Could you check a few things on this model? Use its own coordinates, in mm. A direction names the side the tool comes from. Give positions to 0.01 mm unless a question says otherwise; leave off trailing zeros. Order: outer loops, then holes, each group sorted by start corner. A loop starts at its lowest first (then second) coordinate and runs counter-clockwise, first axis right, second up. Notation, with made-up numbers: (-33, -17.5) -> (-25, -17.5) arc R26 ccw to (-25, -0.5) -> close; hole circle Ø2 at (77, 13.5). An arc over 180 degrees is marked (long way). Answer as CSV lines item,"result". Start each with the question number.
(1) Will these pins go through, and if not, where does the flat tip stop? pin 1 Ø10 at (x, y) = (-2.5, -11) entering from -Z; pin 2 Ø7 at (x, y) = (3, 9.5) entering from +Z; pin 3 Ø3 at (x, y) = (2, -9) entering from -Z; pin 4 Ø1.5 at (x, z) = (0.5, 11.5) entering from -Y.
(2) On a 3-axis mill with a long thin cutter (end or side, diameter ignored), from which of +Z, -Z, +X, -X, +Y, -Y can I reach the whole of each face in a straight line? I mean faces 4 (the face through (-7.75, 8.94, 4.56)), 5 (the face through (0, -11, 8)), 6 (the face through (-11.5, 8.9, 14.6)), 7 (the face through (0.1, -6.5, 15)), 8 (the face through (0, 16, 10)). Say none if no direction works.
(3) I want a section at C-C (z = 12.5). Please give me the cut outline in (x, y).
(4) I want a section at A-A (x = 0). Give the number of separate pieces and of enclosed holes in the cut face, plus the area to 3 significant figures.
(5) We'd pull the mould along X, two halves only. Please class faces 1 (the face through (-12.215, -15.699, 9.874)), 2 (the face through (0, 4.5, 15)), 3 (the face through (0, 0, 0)): released by +X, released by -X, zero draft, split by the parting line, or undercut.
(6) I want a section at D-D (y = -10). Please give me the cut outline in (x, z).
(7) I need wall thicknesses on L1, parallel to Y at x = 2.25, z = 6.5; L2, parallel to Y at x = 7, z = 18.5; L3, parallel to Y at x = 9.5, z = 10.25. Which ranges of each line are inside material? Lowest first, please.
(8) I want a section at B-B (y = 9). Please give me the cut outline in (x, z), plus the area to 3 significant figures.
```python
from build123d import *

# Parameters (mm, degrees)
CROQUIS1_W              = 25
CROQUIS1_H              = 32
SALIENTE_EXTRUIR1_DEPTH = 20
CORTAR_EXTRUIR2_DEPTH   = 20
CORTAR_EXTRUIR3_DEPTH   = 10
CROQUIS9_R              = 2.5
CORTAR_EXTRUIR4_DEPTH   = 10
CROQUIS10_W             = 8
CROQUIS10_H             = 4
CORTAR_EXTRUIR5_DEPTH   = 17
REDONDEO1_R             = 1


with BuildPart() as part:
    # Croquis1 → Saliente-Extruir1 (new body)
    with BuildSketch(Plane.XY):
        Rectangle(CROQUIS1_W, CROQUIS1_H)
    extrude(amount=SALIENTE_EXTRUIR1_DEPTH)

    # Croquis7 → Cortar-Extruir2 (cut)
    with BuildSketch(Plane.XY.offset(20)):
        with BuildLine():
            Line((-5, 11.75), (5, 11.75))
            ThreePointArc((5, 11.75), (7.75, 9), (5, 6.25))
            Line((5, 6.25), (-5, 6.25))
            ThreePointArc((-5, 6.25), (-7.75, 9), (-5, 11.75))
        make_face()
    extrude(amount=-CORTAR_EXTRUIR2_DEPTH, mode=Mode.SUBTRACT)

    # Croquis8 → Cortar-Extruir3 (cut)
    with BuildSketch(Plane.XY.offset(20)):
        with BuildLine():
            Line((-7, 13.5), (7, 13.5))
            ThreePointArc((7, 13.5), (11.5, 9), (7, 4.5))
            Line((7, 4.5), (-7, 4.5))
            ThreePointArc((-7, 4.5), (-11.5, 9), (-7, 13.5))
        make_face()
    extrude(amount=-CORTAR_EXTRUIR3_DEPTH, mode=Mode.SUBTRACT)

    # Croquis9 → Cortar-Extruir4 (cut)
    with BuildSketch(Plane.XZ.offset(16)):
        with Locations(Location((0, 12.5, 0), (0, 0, 270))):
            Circle(CROQUIS9_R)
    extrude(amount=-CORTAR_EXTRUIR4_DEPTH, mode=Mode.SUBTRACT)

    # Croquis10 → Cortar-Extruir5 (cut)
    with BuildSketch(Plane(origin=(0, 0, 0), x_dir=(-1, 0, 0), z_dir=(0, 0, -1))):
        with Locations((0, -9)):
            Rectangle(CROQUIS10_W, CROQUIS10_H)
    extrude(amount=-CORTAR_EXTRUIR5_DEPTH, mode=Mode.SUBTRACT)

    # Redondeo1
    # the kernel refuses this fillet: 1 mm, written as the material it takes off along each edge
    with BuildSketch(Plane(origin=(11.5, -15, 19), x_dir=(0, 0, 1), z_dir=(1, 0, 0))) as redondeo1_piece_1_section:
        Polygon((0, 0), (REDONDEO1_R, 0), (REDONDEO1_R, REDONDEO1_R), (0, REDONDEO1_R), align=None)
    redondeo1_piece_1 = extrude(amount=REDONDEO1_R, mode=Mode.PRIVATE)
    redondeo1_piece_1 = redondeo1_piece_1 - Plane(origin=(11.5, -15, 19), x_dir=(0, 0.7071067811865475, -0.7071067811865475), z_dir=(1, 0, 0)) * Sphere(REDONDEO1_R, mode=Mode.PRIVATE)
    add(redondeo1_piece_1, mode=Mode.SUBTRACT)
    with BuildSketch(Plane(origin=(11.5, 15, 19), x_dir=(1, 0, 0), z_dir=(0, 1, 0))) as redondeo1_piece_2_section:
        Polygon((0, 0), (REDONDEO1_R, 0), (REDONDEO1_R, -REDONDEO1_R), (0, -REDONDEO1_R), align=None)
    redondeo1_piece_2 = extrude(amount=REDONDEO1_R, mode=Mode.PRIVATE)
    redondeo1_piece_2 = redondeo1_piece_2 - Plane(origin=(11.5, 15, 19), x_dir=(-0.7071067811865475, 0, -0.7071067811865475), z_dir=(0, 1, 0)) * Sphere(REDONDEO1_R, mode=Mode.PRIVATE)
    add(redondeo1_piece_2, mode=Mode.SUBTRACT)
    with BuildSketch(Plane(origin=(-11.5, 15, 19), x_dir=(-1, 0, 0), z_dir=(0, 1, 0))) as redondeo1_piece_3_section:
        Polygon((0, 0), (REDONDEO1_R, 0), (REDONDEO1_R, REDONDEO1_R), (0, REDONDEO1_R), align=None)
    redondeo1_piece_3 = extrude(amount=REDONDEO1_R, mode=Mode.PRIVATE)
    redondeo1_piece_3 = redondeo1_piece_3 - Plane(origin=(-11.5, 15, 19), x_dir=(0.7071067811865475, 0, -0.7071067811865475), z_dir=(0, 1, 0)) * Sphere(REDONDEO1_R, mode=Mode.PRIVATE)
    add(redondeo1_piece_3, mode=Mode.SUBTRACT)
    with BuildSketch(Plane(origin=(-11.5, -15, 19), x_dir=(0, 0, 1), z_dir=(-1, 0, 0))) as redondeo1_piece_4_section:
        Polygon((0, 0), (REDONDEO1_R, 0), (REDONDEO1_R, -REDONDEO1_R), (0, -REDONDEO1_R), align=None)
    redondeo1_piece_4 = extrude(amount=REDONDEO1_R, mode=Mode.PRIVATE)
    redondeo1_piece_4 = redondeo1_piece_4 - Plane(origin=(-11.5, -15, 19), x_dir=(0, 0.7071067811865475, -0.7071067811865475), z_dir=(-1, 0, 0)) * Sphere(REDONDEO1_R, mode=Mode.PRIVATE)
    add(redondeo1_piece_4, mode=Mode.SUBTRACT)
    with BuildSketch(Plane(origin=(11.5, 15, 1), x_dir=(1, 0, 0), z_dir=(0, 1, 0))) as redondeo1_piece_5_section:
        Polygon((0, 0), (REDONDEO1_R, 0), (REDONDEO1_R, REDONDEO1_R), (0, REDONDEO1_R), align=None)
    redondeo1_piece_5 = extrude(amount=REDONDEO1_R, mode=Mode.PRIVATE)
    redondeo1_piece_5 = redondeo1_piece_5 - Plane(origin=(11.5, 15, 1), x_dir=(-0.7071067811865475, 0, 0.7071067811865475), z_dir=(0, 1, 0)) * Sphere(REDONDEO1_R, mode=Mode.PRIVATE)
    add(redondeo1_piece_5, mode=Mode.SUBTRACT)
    with BuildSketch(Plane(origin=(-11.5, 15, 1), x_dir=(-1, 0, 0), z_dir=(0, 1, 0))) as redondeo1_piece_6_section:
        Polygon((0, 0), (REDONDEO1_R, 0), (REDONDEO1_R, -REDONDEO1_R), (0, -REDONDEO1_R), align=None)
    redondeo1_piece_6 = extrude(amount=REDONDEO1_R, mode=Mode.PRIVATE)
    redondeo1_piece_6 = redondeo1_piece_6 - Plane(origin=(-11.5, 15, 1), x_dir=(0.7071067811865475, 0, 0.7071067811865475), z_dir=(0, 1, 0)) * Sphere(REDONDEO1_R, mode=Mode.PRIVATE)
    add(redondeo1_piece_6, mode=Mode.SUBTRACT)
    with BuildSketch(Plane(origin=(11.5, -15, 1), x_dir=(0, 0, -1), z_dir=(1, 0, 0))) as redondeo1_piece_7_section:
        Polygon((0, 0), (REDONDEO1_R, 0), (REDONDEO1_R, -REDONDEO1_R), (0, -REDONDEO1_R), align=None)
    redondeo1_piece_7 = extrude(amount=REDONDEO1_R, mode=Mode.PRIVATE)
    redondeo1_piece_7 = redondeo1_piece_7 - Plane(origin=(11.5, -15, 1), x_dir=(0, 0.7071067811865475, 0.7071067811865475), z_dir=(1, 0, 0)) * Sphere(REDONDEO1_R, mode=Mode.PRIVATE)
    add(redondeo1_piece_7, mode=Mode.SUBTRACT)
    with BuildSketch(Plane(origin=(-11.5, -15, 1), x_dir=(0, 0, -1), z_dir=(-1, 0, 0))) as redondeo1_piece_8_section:
        Polygon((0, 0), (REDONDEO1_R, 0), (REDONDEO1_R, REDONDEO1_R), (0, REDONDEO1_R), align=None)
    redondeo1_piece_8 = extrude(amount=REDONDEO1_R, mode=Mode.PRIVATE)
    redondeo1_piece_8 = redondeo1_piece_8 - Plane(origin=(-11.5, -15, 1), x_dir=(0, 0.7071067811865475, 0.7071067811865475), z_dir=(-1, 0, 0)) * Sphere(REDONDEO1_R, mode=Mode.PRIVATE)
    add(redondeo1_piece_8, mode=Mode.SUBTRACT)
    with BuildSketch(Plane(origin=(12.5, -15, 20), x_dir=(0, 0, -1), z_dir=(0, 1, 0)), Plane(origin=(-12.5, 15, 20), x_dir=(0, 0, -1), z_dir=(0, -1, 0))) as redondeo1_piece_9:
        with BuildLine():
            CenterArc((REDONDEO1_R, REDONDEO1_R), REDONDEO1_R, 180, 90)
            Line((0, REDONDEO1_R), (0, 0))
            Line((0, 0), (REDONDEO1_R, 0))
        make_face()
    extrude(amount=30, mode=Mode.SUBTRACT)
    with BuildSketch(Plane(origin=(11.5, 16, 20), x_dir=(0, 0, -1), z_dir=(-1, 0, 0)), Plane(origin=(-11.5, -16, 0), x_dir=(0, 1, 0), z_dir=(1, 0, 0))) as redondeo1_piece_10:
        with BuildLine():
            CenterArc((REDONDEO1_R, REDONDEO1_R), REDONDEO1_R, 180, 90)
            Line((0, REDONDEO1_R), (0, 0))
            Line((0, 0), (REDONDEO1_R, 0))
        make_face()
    extrude(amount=23, mode=Mode.SUBTRACT)
    with BuildSketch(Plane(origin=(5, 6.25, 10), x_dir=(0, 0, -1), z_dir=(-1, 0, 0)), Plane(origin=(-5, 11.75, 10), x_dir=(0, 0, -1), z_dir=(1, 0, 0))) as redondeo1_piece_11:
        with BuildLine():
            CenterArc((REDONDEO1_R, REDONDEO1_R), REDONDEO1_R, 180, 90)
            Line((0, REDONDEO1_R), (0, 0))
            Line((0, 0), (REDONDEO1_R, 0))
        make_face()
    extrude(amount=10, mode=Mode.SUBTRACT)
    with BuildSketch(Plane(origin=(-7, 9, 20), x_dir=(0, -1, 0), z_dir=(1, 0, 0))) as redondeo1_piece_12:
        with BuildLine():
            CenterArc((4.5 + REDONDEO1_R, REDONDEO1_R), REDONDEO1_R, 180, 90)
            Line((4.5, REDONDEO1_R), (4.5, 0))
            Line((4.5, 0), (4.5 + REDONDEO1_R, 0))
        make_face()
    revolve(axis=Axis((-7, 9, 20), (0, 0, -1)), revolution_arc=180, mode=Mode.SUBTRACT)
    with BuildSketch(Plane(origin=(7, 4.5, 20), x_dir=(0, -1, 0), z_dir=(-1, 0, 0)), Plane(origin=(-7, 13.5, 20), x_dir=(0, 1, 0), z_dir=(1, 0, 0))) as redondeo1_piece_13:
        with BuildLine():
            CenterArc((REDONDEO1_R, -REDONDEO1_R), REDONDEO1_R, 90, 90)
            Line((0, -REDONDEO1_R), (0, 0))
            Line((0, 0), (REDONDEO1_R, 0))
        make_face()
    extrude(amount=14, mode=Mode.SUBTRACT)
    with BuildSketch(Plane(origin=(7, 9, 20), x_dir=(0, 1, 0), z_dir=(-1, 0, 0))) as redondeo1_piece_14:
        with BuildLine():
            CenterArc((4.5 + REDONDEO1_R, REDONDEO1_R), REDONDEO1_R, 180, 90)
            Line((4.5, REDONDEO1_R), (4.5, 0))
            Line((4.5, 0), (4.5 + REDONDEO1_R, 0))
        make_face()
    revolve(axis=Axis((7, 9, 20), (0, 0, -1)), revolution_arc=180, mode=Mode.SUBTRACT)
    with BuildSketch(Plane(origin=(-5, 9, 10), x_dir=(0, 1, 0), z_dir=(1, 0, 0))) as redondeo1_piece_15:
        with BuildLine():
            CenterArc((2.75 + REDONDEO1_R, -REDONDEO1_R), REDONDEO1_R, 90, 90)
            Line((2.75 + REDONDEO1_R, 0), (2.75, 0))
            Line((2.75, 0), (2.75, -REDONDEO1_R))
        make_face()
    revolve(axis=Axis((-5, 9, 10), (0, 0, 1)), revolution_arc=180, mode=Mode.SUBTRACT)
    with BuildSketch(Plane(origin=(5, 9, 10), x_dir=(0, -1, 0), z_dir=(-1, 0, 0))) as redondeo1_piece_16:
        with BuildLine():
            CenterArc((2.75 + REDONDEO1_R, -REDONDEO1_R), REDONDEO1_R, 90, 90)
            Line((2.75 + REDONDEO1_R, 0), (2.75, 0))
            Line((2.75, 0), (2.75, -REDONDEO1_R))
        make_face()
    revolve(axis=Axis((5, 9, 10), (0, 0, 1)), revolution_arc=180, mode=Mode.SUBTRACT)
    with BuildSketch(Plane(origin=(11.5, 16, 0), x_dir=(0, 0, 1), z_dir=(-1, 0, 0)), Plane(origin=(-11.5, -16, 20), x_dir=(0, 1, 0), z_dir=(1, 0, 0))) as redondeo1_piece_17:
        with BuildLine():
            CenterArc((REDONDEO1_R, -REDONDEO1_R), REDONDEO1_R, 90, 90)
            Line((0, -REDONDEO1_R), (0, 0))
            Line((0, 0), (REDONDEO1_R, 0))
        make_face()
    extrude(amount=23, mode=Mode.SUBTRACT)
    with BuildSketch(Plane(origin=(0, -16, 12.5), x_dir=(0, 0, -1), z_dir=(-1, 0, 0))) as redondeo1_piece_18:
        with BuildLine():
            CenterArc((2.5 + REDONDEO1_R, -REDONDEO1_R), REDONDEO1_R, 90, 90)
            Line((2.5, -REDONDEO1_R), (2.5, 0))
            Line((2.5, 0), (2.5 + REDONDEO1_R, 0))
        make_face()
    revolve(axis=Axis((0, -16, 12.5), (0, -1, 0)), mode=Mode.SUBTRACT)
    with BuildSketch(Plane(origin=(12.5, -15, 0), x_dir=(0, 0, 1), z_dir=(0, 1, 0)), Plane(origin=(-12.5, 15, 0), x_dir=(0, 0, 1), z_dir=(0, -1, 0))) as redondeo1_piece_19:
        with BuildLine():
            CenterArc((REDONDEO1_R, -REDONDEO1_R), REDONDEO1_R, 90, 90)
            Line((0, -REDONDEO1_R), (0, 0))
            Line((0, 0), (REDONDEO1_R, 0))
        make_face()
    extrude(amount=30, mode=Mode.SUBTRACT)
    with BuildSketch(Plane(origin=(-12.5, 16, 1), x_dir=(1, 0, 0), z_dir=(0, 0, 1)), Plane(origin=(-12.5, -16, 1), x_dir=(0, 1, 0), z_dir=(0, 0, 1))) as redondeo1_piece_20:
        with BuildLine():
            CenterArc((REDONDEO1_R, -REDONDEO1_R), REDONDEO1_R, 90, 90)
            Line((0, -REDONDEO1_R), (0, 0))
            Line((0, 0), (REDONDEO1_R, 0))
        make_face()
    extrude(amount=18, mode=Mode.SUBTRACT)
    with BuildSketch(Plane(origin=(12.5, 16, 1), x_dir=(-1, 0, 0), z_dir=(0, 0, 1)), Plane(origin=(12.5, -16, 1), x_dir=(0, 1, 0), z_dir=(0, 0, 1))) as redondeo1_piece_21:
        with BuildLine():
            CenterArc((REDONDEO1_R, REDONDEO1_R), REDONDEO1_R, 180, 90)
            Line((0, REDONDEO1_R), (0, 0))
            Line((0, 0), (REDONDEO1_R, 0))
        make_face()
    extrude(amount=18, mode=Mode.SUBTRACT)


solid = part.part
```
Final values:
1,pin 1,"z = 0"
1,pin 2,"z = 10"
1,pin 3,"z = 17"
1,pin 4,"y = -6"
2,face 4,"+Z, -Z"
2,face 5,"-Z"
2,face 6,"+Z"
2,face 7,"-Y"
2,face 8,"+Z, -Z, +X, -X, +Y"
3,outline,"(-12.5, -15) arc R1 ccw to (-11.5, -16) -> (-3.5, -16) arc R1 ccw to (-2.5, -15) -> (-2.5, -11) -> (-4, -11) -> (-4, -7) -> (-2.5, -7) -> (-2.5, -6) -> (2.5, -6) -> (2.5, -7) -> (4, -7) -> (4, -11) -> (2.5, -11) -> (2.5, -15) arc R1 ccw to (3.5, -16) -> (11.5, -16) arc R1 ccw to (12.5, -15) -> (12.5, 15) arc R1 ccw to (11.5, 16) -> (-11.5, 16) arc R1 ccw to (-12.5, 15) -> close; hole (-7, 4.5) -> (7, 4.5) arc R4.5 ccw to (7, 13.5) -> (-7, 13.5) arc R4.5 ccw to start"
4,separate pieces,"3"
4,enclosed holes,"0"
4,area,"395 mm²"
5,face 1,"released by -X"
5,face 2,"undercut"
5,face 3,"zero draft"
6,outline,"(-12.5, 1) arc R1 ccw to (-11.5, 0) -> (-4, 0) -> (-4, 17) -> (4, 17) -> (4, 0) -> (11.5, 0) arc R1 ccw to (12.5, 1) -> (12.5, 19) arc R1 ccw to (11.5, 20) -> (-11.5, 20) arc R1 ccw to (-12.5, 19) -> close"
7,L1,"-16 to -11, -7 to 6.25, 11.75 to 16"
7,L2,"-16 to 4.5, 13.5 to 16"
7,L3,"-16 to 5.26, 12.74 to 16"
8,outline,"(-12.5, 1) arc R1 ccw to (-11.5, 0) -> (-7.75, 0) -> (-7.75, 9) arc R1 ccw to (-8.75, 10) -> (-11.5, 10) -> (-11.5, 19) arc R1 ccw to (-12, 19.87) arc R1 ccw to (-12.5, 19) -> close; (7.75, 0) -> (11.5, 0) arc R1 ccw to (12.5, 1) -> (12.5, 19) arc R1 ccw to (12, 19.87) arc R1 ccw to (11.5, 19) -> (11.5, 10) -> (8.75, 10) arc R1 ccw to (7.75, 9) -> close"
8,area,"113 mm²"
